Here's how the part is built. I have some questions about the finished solid (model axes, mm). Coordinates: 2 decimals unless noted, no trailing zeros. Order: outer loops, then holes, each group sorted by start corner. A loop starts at its lowest first (then second) coordinate and runs counter-clockwise, first axis right, second up. Notation, with made-up numbers: (-40, -25) - (-12, -25) arc R17 ccw to (-12, -12) - close; hole circle Ø3 at (-0.75, 23.25). An arc over 180 degrees is marked (long way). Answer in a Markdown table with one row per item. Add a question column.
Item 1: If I drill on line 1 along Y through (x, z) = (0, 12.5); line 2 along X through (y, z) = (-474.5, 5.5); line 3 along Y through (x, z) = (-111, 6), over which ranges is the centre line in solid material (lowest first)? Write a range as from..to.
Item 2: I want a section at D-D (x = 551). Please give me the cut outline in (y, z) (3 decimals), plus the area to 3 significant figures.
Item 3: I want a section at C-C (x = 0). Please give me the cut outline in (y, z) (3 decimals), plus the area to 3 significant figures.
Item 4: Will these pins go through, and if not, where does the flat tip stop? pin 1 Ø8 at (x, y) = (168.5, -482) entering from -Z; pin 2 Ø10 at (x, z) = (279, 13.5) entering from -Y.
Item 5: I want a section at A-A (y = 0). Please give me the cut outline in (x, z) (3 decimals).
Item 6: I want a section at B-B (z = 7). Please give me the cut outline in (x, y).
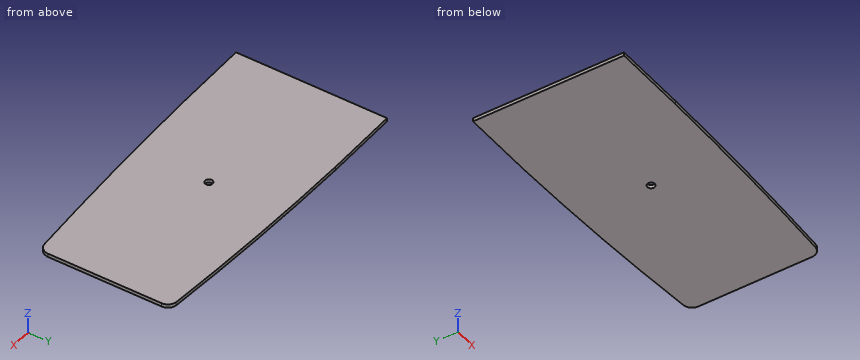
```python
from build123d import *

# Parameters (mm, degrees)
F0_R     = 30.226
F1_DEPTH = 28.575


with BuildPart() as f1:
    # F0 (on Top) → F1 (new body)
    with BuildSketch(Plane.XY):
        with BuildLine():
            Line((1219.2, -470.965787), (1219.2, 445.565831))
            ThreePointArc((1219.2, 445.565831), (1201.198829, 494.752581), (1155.700359, 520.699984))
            Line((1155.700359, 520.699984), (-1219.2, 609.6))
            Line((-1219.2, 609.6), (-1219.2, -609.6))
            Line((-1219.2, -609.6), (1155.7, -546.1))
            ThreePointArc((1155.7, -546.1), (1201.198711, -520.152675), (1219.2, -470.965787))
        make_face()
        Circle(F0_R, mode=Mode.SUBTRACT)
        with BuildLine():
            Line((-1219.2, 609.6), (1155.700359, 520.699984))
            ThreePointArc((1155.700359, 520.699984), (273.88184, 581.6644), (-609.6, 609.6))
            Line((-609.6, 609.6), (-1219.2, 609.6))
        make_face()
        with BuildLine():
            ThreePointArc((-609.6, -609.6), (273.474389, -589.648025), (1155.7, -546.1))
            Line((1155.7, -546.1), (-1219.2, -609.6))
            Line((-1219.2, -609.6), (-609.6, -609.6))
        make_face()
    extrude(amount=F1_DEPTH)


solid = f1.part
```
Values follow:
| question | item | result |
|---|---|---|
| 1 | line 1 | y = -598.35..-30.23, 30.23..593.86 |
| 1 | line 2 | x = -1219.2..1219.12 |
| 1 | line 3 | y = -601.24..597.9 |
| 2 | outline | (-578.497, 0) - (566.076, 0) - (566.076, 28.575) - (-578.497, 28.575) - close |
| 2 | area | 32,700 mm^2 |
| 3 | outline | (-598.352, 0) - (-30.226, 0) - (-30.226, 28.575) - (-598.352, 28.575) - close; (30.226, 0) - (593.864, 0) - (593.864, 28.575) - (30.226, 28.575) - close |
| 3 | area | 32,300 mm^2 |
| 4 | pin 1 | stops at z = 0 |
| 4 | pin 2 | stops at y = -589.63 |
| 5 | outline | (-1219.2, 0) - (-30.226, 0) - (-30.226, 28.575) - (-1219.2, 28.575) - close; (30.226, 0) - (1219.2, 0) - (1219.2, 28.575) - (30.226, 28.575) - close |
| 6 | outline | (-1219.2, -609.6) - (-609.6, -609.6) arc R33044.27 ccw to (1155.7, -546.1) arc R76.2 ccw to (1219.2, -470.97) - (1219.2, 445.57) arc R76.2 ccw to (1155.7, 520.7) arc R23625.78 ccw to (-609.6, 609.6) - (-1219.2, 609.6) - close; hole circle Ø60.45 at (0, 0) |
